Check sheet for the modelled part. Datum: model origin and axes. Units: mm. A direction names the side the tool comes from. Coordinates: 2 decimals unless noted, no trailing zeros. Order: outer loops, then holes, each group sorted by start corner. A loop starts at its lowest first (then second) coordinate and runs counter-clockwise, first axis right, second up.
1. Cross-section at A-A (y = 1.5). Enter the section's corners in (x, z), then the cut area to 3 significant figures.
2. Set-up check for faces 1 (the flat face through (2, 10, 0)), 2 (the cylindrical face through (-0.54, 10.15, -2.44)): record each of +Z, -Z, +X, -X, +Y, -Y from which the full face is reachable in a straight line by a thin tool's end or side.
3. Gauge pin test, flat end, axial feed: pin 1 Ø3 at (x, y) = (-1, 6.5) entering from -Z. Record the tip position at first contact, or that the pin passes through.
4. Thickness scan on line 1 (X direction, y = 2, z = -0.9); line 2 (Z direction, x = 0.4, y = 6.25). Record the ranges inside material, lowest first.
Autodesk Inventor part; units mm, degrees
ref_plane "YZ Plane" through (0, 0, 0) normal (1, 0, 0) x (0, 1, 0)
ref_plane "XZ Plane" through (0, 0, 0) normal (0, 1, 0) x (-1, 0, 0)
ref_plane "XY Plane" through (0, 0, 0) normal (0, 0, 1) x (1, 0, 0)
sketch "Sketch1" plane through (0, 0, 0) normal (0, 1, 0) x (-1, 0, 0)
  circle A0 centre (0, 0) radius 1.5
  dimension "d0" = 3
extrude "Extrusion1" add sketch "Sketch1" along normal blind 10
sketch "Sketch2" plane through (0, 10, 0) normal (0, 1, 0) x (1, 0, 0)
  circle A0 centre (0, 0) radius 2.5
  dimension "d3" = 5
extrude "Extrusion2" add sketch "Sketch2" along normal blind 2
fillet "Fillet1" radius 1.7 1 edges at (-2.5, 12, 0)
chamfer "Chamfer1" distance 0.3 angle 45 1 edges at (1.5, 0, 0)
thread "Thread1"
properties part number "M3x10 Screw Steel" material "Stainless Steel"
Data:
1. outline: circle Ø3 at (0, 0)
1. area: 7.07 mm2
2. face 1: -Y
2. face 2: +Y, -Y
3. pin 1: stops at z = -1.5
4. line 1: x = -1.2 to 1.2
4. line 2: z = -1.45 to 1.45
